```python
from build123d import *

# Parameters (mm, degrees)
F0_W     = 2032
F0_H     = 1016
F1_DEPTH = 720
F3_DEPTH = 3810
F5_DEPTH = 1143


with BuildPart() as f1:
    # F0 (on Top) → F1 (new body)
    with BuildSketch(Plane.XY):
        with Locations((1016, 508)):
            Rectangle(F0_W, F0_H)
    extrude(amount=F1_DEPTH)

    # F2 (on face) → F3 (cut)
    with BuildSketch(Plane.YZ.offset(2032)):
        Polygon((76.199963, 0.074586), (76.188638, 0), (101.6, 0), (924.743533, 0), (940.272614, 0), (838.2, 669.2), (177.8, 669.2), align=None)
        Polygon((101.6, 669.2), (0, 669.2), (0, 0), align=None)
        Polygon((1016, 0), (1016, 669.2), (914.4, 669.2), align=None)
    extrude(amount=-F3_DEPTH, mode=Mode.SUBTRACT)

    # F4 (on Front) → F5 (cut)
    with BuildSketch(Plane.XZ):
        Polygon((415.1, 0), (2584.981293, 0), (2584.981301, 666.419255), (415.1, 666.419255), align=None)
        Polygon((250, 666.419255), (0, 666.419255), (0, 0), (338.9, 0), align=None)
        Polygon((3000.081301, 0), (3000.081301, 666.419255), (2750.081301, 666.419255), (2661.181293, 0), (2740.58795, 0), align=None)
    extrude(amount=-F5_DEPTH, mode=Mode.SUBTRACT)


solid = f1.part
```
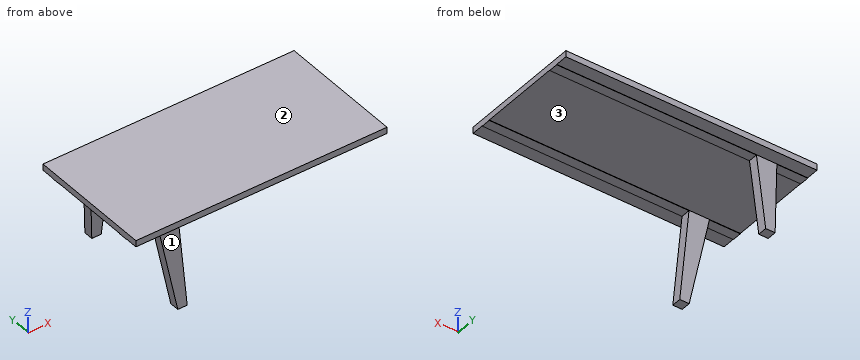
Input: part model. Units: mm. Frame: model coordinates. Face numbers are marked on the shaded views. Give positions to 0.01 mm unless a question says otherwise; leave off trailing zeros. Order: outer loops, then holes, each group sorted by start corner. A loop starts at its lowest first (then second) coordinate and runs counter-clockwise, first axis right, second up.
1. Pin query (flat end, axial travel): pin 1 Ø12 at (y, z) = (881, 605.5) entering from +X; pin 2 Ø4 at (x, y) = (332, 444) entering from -Z. Return the tip coordinate at first contact, or that it passes through.
Computed:
pin 1: stops at x = 415.1
pin 2: stops at z = 669.2
2. Cut plane A-A (z = 287.5). Return loops of the section in (x, y), and give its area (3 significant figures).
Computed:
outline: (300.55, 43.65) - (415.1, 43.65) - (415.1, 119.84) - (300.55, 119.84) - close; (300.55, 896.42) - (415.1, 896.42) - (415.1, 972.35) - (300.55, 972.35) - close
area: 17,400 mm2
3. Cut plane D-D (z = 429.5). Return loops of the section in (x, y).
Computed:
outline: (281.6, 65.21) - (415.1, 65.21) - (415.1, 141.4) - (281.6, 141.4) - close; (281.6, 874.76) - (415.1, 874.76) - (415.1, 950.79) - (281.6, 950.79) - close
4. Line query: probe 1 along Z at (x, y) = (1513.5, 771.5); probe 2 along Z at (x, y) = (635, 858.5); probe 3 along Y at (x, z) = (275.5, 563). Output: solid intervals per line, ascending.
Computed:
probe 1: z = 669.2 to 720
probe 2: z = 666.42 to 720
probe 3: y = 85.48 to 161.67, 854.4 to 930.52
5. Cut plane B-B (x = 1185.5). Return loops of the section in (y, z), and give its area (3 significant figures).
Computed:
outline: (0, 669.2) - (101.6, 669.2) - (101.18, 666.42) - (177.38, 666.42) - (177.8, 669.2) - (838.2, 669.2) - (838.62, 666.42) - (914.82, 666.42) - (914.4, 669.2) - (1016, 669.2) - (1016, 720) - (0, 720) - close
area: 52,000 mm2
6. Cut plane C-C (y = 646). Return loops of the section in (x, z), and give its area (3 significant figures).
Computed:
outline: (0, 669.2) - (2032, 669.2) - (2032, 720) - (0, 720) - close
area: 103,000 mm2
7. Draft query along Z for the marked faces 1, 2 and 3. Return one class per face: released by +Z, released by -Z, zero draft, split by the parting line, or undercut.
Computed:
face 1: undercut
face 2: released by +Z
face 3: released by -Z
